Read the model definition and answer for the solid it produces. Units are mm, in the model's axes. A direction names the side the tool comes from. Give positions to 0.01 mm unless a question says otherwise; leave off trailing zeros. Write each loop counter-clockwise with the first axis right and the second up, starting at its lowest first coordinate (ties: lowest second). Pieces come first, ordered by that corner, then holes. Notation, with made-up numbers: (-29.75, 54) - (-20.75, 54) arc R21 cw to (-20.75, 66) - close; hole circle Ø8 at (31.25, -13). An arc over 180 degrees is marked (long way). Answer as CSV lines item,"result".
```python
from build123d import *

# Parameters (mm, degrees)
ESQUISSE1_W        = 30
ESQUISSE1_H        = 26
ESQUISSE1_R        = 1.05
ESQUISSE1_W_2      = 15
ESQUISSE1_H_2      = 20.5
BOSS_EXTRU_1_DEPTH = 3
CONG_1_R           = 2.5
ESQUISSE3_R        = 1.75
BOSS_EXTRU_3_DEPTH = 5


with BuildPart() as part:
    # Esquisse1 → Boss.-Extru.1 (new body)
    with BuildSketch(Plane.XY):
        Rectangle(ESQUISSE1_W, ESQUISSE1_H)
        with Locations((-10.5, 2.638)):
            Circle(ESQUISSE1_R, mode=Mode.SUBTRACT)
        with Locations((10.5, 2.638)):
            Circle(ESQUISSE1_R, mode=Mode.SUBTRACT)
        with Locations((-10.5, -9.862)):
            Circle(ESQUISSE1_R, mode=Mode.SUBTRACT)
        with Locations((10.5, -9.862)):
            Circle(ESQUISSE1_R, mode=Mode.SUBTRACT)
        with Locations((0, -0.25)):
            Rectangle(ESQUISSE1_W_2, ESQUISSE1_H_2, mode=Mode.SUBTRACT)
    extrude(amount=BOSS_EXTRU_1_DEPTH)

    # Congé1
    cong_1_edges = [part.edges().sort_by_distance(p)[0] for p in [
        (15, 13, 1.5),
        (-15, 13, 1.5),
    ]]
    fillet(cong_1_edges, radius=CONG_1_R)

    # Esquisse3 → Boss.-Extru.3 (add)
    with BuildSketch(Plane(origin=(15, 0, 0), x_dir=(0, 0, -1), z_dir=(1, 0, 0))):
        with BuildLine():
            ThreePointArc((-3, -11.5), (-7.203775615, -17.605699404), (0, -19.354101966))
            Line((0, -19.354101966), (0, -13))
            Line((0, -13), (-3, -13))
            Line((-3, -13), (-3, -11.5))
        make_face()
        with Locations(Location((-3, -16, 0), (0, 0, 90))):
            Circle(ESQUISSE3_R, mode=Mode.SUBTRACT)
    boss_extru_3 = extrude(amount=-BOSS_EXTRU_3_DEPTH)

    # Symétrie2: Boss.-Extru.3 across plane
    add(boss_extru_3.mirror(Plane(origin=(0, 0, 0), x_dir=(0, 0, 1), z_dir=(1, 0, 0))))


solid = part.part
```
(1) For faces 4 (the cylindrical face through (-12.535, -14.383, 2.33)), 5 (the flat face through (0, -13, 1)), 6 (the flat face through (0, 10, 1)), determine the directions among +Z, -Z, +X, -X, +Y, -Y from which every point of the face is accessible in a straight line to the end or side of a thin tool.
Worked out:
face 4,"+X, -X"
face 5,"+Z, -Z, -Y"
face 6,"+Z, -Z"
(2) A cutting plane is placed at C-C (x = 0). Write down the section's boundary in (y, z).
Worked out:
outline,"(-13, 0) - (-10.5, 0) - (-10.5, 3) - (-13, 3) - close; (10, 0) - (13, 0) - (13, 3) - (10, 3) - close"
(3) A cutting plane is placed at A-A (x = 10.5). Write down the section's boundary in (y, z), and give its area (3 significant figures).
Worked out:
outline,"(-19.35, 0) - (-10.91, 0) - (-10.91, 3) - (-11.5, 3) arc R4.5 ccw (long way) to start; (-8.81, 0) - (1.59, 0) - (1.59, 3) - (-8.81, 3) - close; (3.69, 0) - (13, 0) - (13, 3) - (3.69, 3) - close; hole circle Ø3.5 at (-16, 3)"
area,"109 mm^2"
(4) Find the intervals of material crossed by L1, parallel to X at y = -17, z = 1.5; L2, parallel to X at y = 7, z = 2.75; L3, parallel to Z at x = 13.15, y = -16, in increasing order.
Worked out:
L1,"x = -15 to -10, 10 to 15"
L2,"x = -15 to -7.5, 7.5 to 15"
L3,"z = 0 to 1.25, 4.75 to 7.5"
(5) A cutting plane is placed at B-B (y = 0). Write down the section's boundary in (x, z).
Worked out:
outline,"(-15, 0) - (-7.5, 0) - (-7.5, 3) - (-15, 3) - close; (7.5, 0) - (15, 0) - (15, 3) - (7.5, 3) - close"
(6) A cutting plane is placed at D-D (z = 2.5). Write down the section's boundary in (x, y), and give its area (3 significant figures).
Worked out:
outline,"(-15, -20.47) - (-10, -20.47) - (-10, -17.68) - (-15, -17.68) - close; (-15, -14.32) - (-10, -14.32) - (-10, -13) - (10, -13) - (10, -14.32) - (15, -14.32) - (15, 10.5) arc R2.5 ccw to (12.5, 13) - (-12.5, 13) arc R2.5 ccw to (-15, 10.5) - close; (10, -20.47) - (15, -20.47) - (15, -17.68) - (10, -17.68) - close; hole circle Ø2.1 at (-10.5, -9.86); hole circle Ø2.1 at (-10.5, 2.64); hole (-7.5, -10.5) - (7.5, -10.5) - (7.5, 10) - (-7.5, 10) - close; hole circle Ø2.1 at (10.5, -9.86); hole circle Ø2.1 at (10.5, 2.64)"
area,"497 mm^2"
(7) The mould has two halves that part along Z. Classify faces 1 (the cylindrical face through (12.535, -17.491, 7.246)), 2 (the flat face through (10, -17, 5)), 3 (the cylindrical face through (12.535, -14.383, 2.33)): +Z half, -Z half, draft (parallel to the pull), parting line (faces both ways), or undercut.
Worked out:
face 1,"parting line"
face 2,"draft"
face 3,"undercut"
(8) Each of these flat-tipped pins is pushed along its axis until it touches: P1, Ø1.5, axis at x = 1, z = 1, coming from the -Y side; P2, Ø6, axis at x = -6, y = 8, coming from the -Z side; P3, Ø2, axis at y = -16, z = 3, coming from the +X side; P4, Ø2, axis at x = 10.5, z = 6, coming from the +Y side. Where does it stop, or does it pass through?
Worked out:
P1,"stops at y = -13"
P2,"stops at z = 0"
P3,"passes through"
P4,"stops at y = -11.97"
